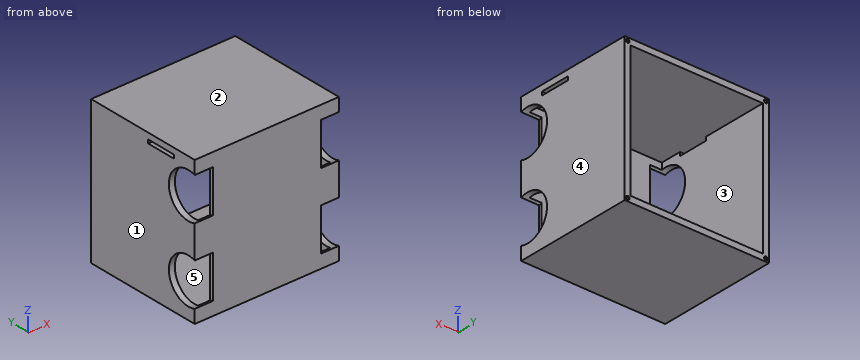
```python
from build123d import *

# Parameters (mm, degrees)
SKETCH2_W               = 240
SKETCH2_H               = 240
BOSS_EXTRUDE1_DEPTH     = 200
SKETCH17_W              = 220
SKETCH17_H              = 220
CUT_EXTRUDE1_DEPTH      = 195
SKETCH20_R              = 37.5
CUT_EXTRUDE3_DEPTH      = 30
SKETCH21_R              = 37.5
CUT_EXTRUDE4_DEPTH      = 30
SKETCH22_R              = 3
CUT_EXTRUDE5_DEPTH      = 2
SKETCH24_W              = 6
SKETCH24_H              = 50
CUT_EXTRUDE7_DEPTH      = 1
CUT_EXTRUDE7_DEPTH_BACK = 241


with BuildPart() as part:
    # Sketch2 → Boss-Extrude1 (new body)
    with BuildSketch(Plane(origin=(0, -113.102021597, 0), x_dir=(1, 0, 0), z_dir=(0, 1, 0))):
        Rectangle(SKETCH2_W, SKETCH2_H)
    extrude(amount=BOSS_EXTRUDE1_DEPTH)

    # Sketch17 → Cut-Extrude1 (cut)
    with BuildSketch(Plane(origin=(0, 86.897978403, 0), x_dir=(1, 0, 0), z_dir=(0, 1, 0))):
        Rectangle(SKETCH17_W, SKETCH17_H)
    extrude(amount=-CUT_EXTRUDE1_DEPTH, mode=Mode.SUBTRACT)

    # Sketch20 → Cut-Extrude3 (cut)
    with BuildSketch(Plane(origin=(120, 0, 0), x_dir=(0, 0, -1), z_dir=(1, 0, 0))):
        with Locations((-62.5, -100.602021597)):
            Circle(SKETCH20_R)
        with Locations((62.5, -100.602021597)):
            Circle(SKETCH20_R)
    extrude(amount=-CUT_EXTRUDE3_DEPTH, mode=Mode.SUBTRACT)

    # Sketch21 → Cut-Extrude4 (cut)
    with BuildSketch(Plane.ZY.offset(120)):
        with Locations((62.5, -100.602021597)):
            Circle(SKETCH21_R)
        with Locations((-62.5, -100.602021597)):
            Circle(SKETCH21_R)
    extrude(amount=-CUT_EXTRUDE4_DEPTH, mode=Mode.SUBTRACT)

    # Sketch22 → Cut-Extrude5 (cut)
    with BuildSketch(Plane(origin=(0, 86.897978403, 0), x_dir=(1, 0, 0), z_dir=(0, 1, 0))):
        with Locations((-115, 115)):
            Circle(SKETCH22_R)
        with Locations((-115, -115)):
            Circle(SKETCH22_R)
        with Locations((115, -115)):
            Circle(SKETCH22_R)
        with Locations((115, 115)):
            Circle(SKETCH22_R)
    extrude(amount=-CUT_EXTRUDE5_DEPTH, mode=Mode.SUBTRACT)

    # Sketch24 → Cut-Extrude7 (cut, two sides)
    with BuildSketch(Plane.ZY.offset(120)) as cut_extrude7_sk:
        with Locations((107, -48.102021597)):
            Rectangle(SKETCH24_W, SKETCH24_H)
    extrude(amount=CUT_EXTRUDE7_DEPTH, mode=Mode.SUBTRACT)
    extrude(cut_extrude7_sk.sketch, amount=-CUT_EXTRUDE7_DEPTH_BACK, mode=Mode.SUBTRACT)


solid = part.part
```
Geometry check sheet. Reference: the model listing, model coordinates, mm. Face numbers are marked on the shaded views. A direction names the side the tool comes from. Coordinates: 2 decimals unless noted, no trailing zeros. Order: outer loops, then holes, each group sorted by start corner. A loop starts at its lowest first (then second) coordinate and runs counter-clockwise, first axis right, second up.
Item 1: Mould release check, pull along Z, two halves, no side actions. Record for the marked faces 1, 2 and 3: released by +Z, released by -Z, zero draft, split by the parting line, or undercut.
Item 2: Section check D-D (y = -80). Enter the section's corners in (x, z).
Item 3: Section check A-A (z = -62.5). Enter the section's corners in (x, y).
Item 4: Depth check by flat-ended pin: pin 1 (8 mm diameter, centred on x = -65, z = -94.5, fed in from +Y); pin 2 (1.5 mm diameter, centred on y = -111.5, z = -80, fed in from +X); pin 3 (4 mm diameter, centred on y = -110.5, z = -44.5, fed in from -X). Enter the tip coordinate at first touch or a pass-through.
Item 5: Section check C-C (x = 40.5). Enter the section's corners in (y, z), plus the area to 3 significant figures.
Item 6: Scan lines: line 1 along Z through (x, y) = (115, 85.8); line 2 along X through (y, z) = (-14.5, 57). Record each from-to range of solid material in increasing order.
Item 7: Tool access check on the marked faces 4 and 5. Record the directions out of +Z, -Z, +X, -X, +Y, -Y that give a thin tool (end or side, any length) a straight path to the whole face; none if there is none.
Item 8: Section check B-B (y = -8.5). Enter the section's corners in (x, z).
Check sheet entries:
1. face 1: zero draft
1. face 2: released by +Z
1. face 3: undercut
2. outline: (-120, -120) - (120, -120) - (120, -93.83) - (110, -93.83) - (110, -110) - (-110, -110) - (-110, -93.83) - (-120, -93.83) - close; (-120, -31.17) - (-110, -31.17) - (-110, 31.17) - (-120, 31.17) - close; (-120, 93.83) - (-110, 93.83) - (-110, 110) - (110, 110) - (110, 93.83) - (120, 93.83) - (120, 120) - (-120, 120) - close; (110, -31.17) - (120, -31.17) - (120, 31.17) - (110, 31.17) - close
3. outline: (-120, -63.1) - (-110, -63.1) - (-110, 86.9) - (-120, 86.9) - close; (-90, -113.1) - (90, -113.1) - (90, -108.1) - (-90, -108.1) - close; (110, -63.1) - (120, -63.1) - (120, 86.9) - (110, 86.9) - close
4. pin 1: stops at y = -108.1
4. pin 2: stops at x = 90
4. pin 3: stops at x = -90
5. outline: (-113.1, -120) - (86.9, -120) - (86.9, -110) - (-108.1, -110) - (-108.1, 110) - (86.9, 110) - (86.9, 120) - (-113.1, 120) - close
5. area: 5,100 mm2
6. line 1: z = -120 to -118, -112 to 112, 118 to 120
6. line 2: x = -120 to -110, 110 to 120
7. face 4: +Z, -Z, +X, +Y, -Y
7. face 5: +Y
8. outline: (-120, -120) - (120, -120) - (120, 120) - (-120, 120) - close; hole (-110, -110) - (110, -110) - (110, 110) - (-110, 110) - close
